from build123d import *

# Parameters (mm, degrees)
IZIM1_W                          = 400
IZIM1_H                          = 400
Y_KSEKLIK_EKSTR_ZYON1_DEPTH      = 30
F_25_5_25_5_AP_DELIK1_AT_2_COUNT = 2
F_25_5_25_5_AP_DELIK1_AT_2_PITCH = 280
F_25_5_25_5_AP_DELIK1_AT_3_COUNT = 2
F_25_5_25_5_AP_DELIK1_AT_3_PITCH = 280
F_25_5_25_5_AP_DELIK1_AT_4_COUNT = 2
F_25_5_25_5_AP_DELIK1_AT_4_PITCH = 395.979797464
KES_EKSTR_ZYON3_DEPTH            = 30
M12_SHCS_IN_HAV_A1_D             = 13
M12_SHCS_IN_HAV_A1_CBORE_D       = 20
M12_SHCS_IN_HAV_A1_CBORE_DEPTH   = 12
M14X2_0_DI_LI_DELIK1_D           = 12
M14X2_0_DI_LI_DELIK1_DEPTH       = 20
M14X2_0_DI_LI_DELIK1_TIP         = 3.605163714


with BuildPart() as part:
    # Çizim1 → Yükseklik-Ekstrüzyon1 (new body)
    with BuildSketch(Plane(origin=(0, 0, 0), x_dir=(1, 0, 0), z_dir=(0, 1, 0))):
        Rectangle(IZIM1_W, IZIM1_H)
    extrude(amount=Y_KSEKLIK_EKSTR_ZYON1_DEPTH)

    # Çizim3 → Ø25.5 (25.5) Çap Delik1 (revolve, cut)
    with BuildSketch(Plane(origin=(-140, 30, 140), x_dir=(0, 0, 1), z_dir=(1, 0, 0))):
        Polygon((0, 0), (0, 30), (20, 30), (12.75, 22.75), (12.75, 7.25), (20, 0), align=None)
    f_25_5_25_5_ap_delik1 = revolve(axis=Axis((-140, 36.35, 140), (0, -1, 0)), mode=Mode.SUBTRACT)

    # Ø25.5 (25.5) Çap Delik1 at 2: Ø25.5 (25.5) Çap Delik1 ×2
    with Locations(*[(0, 0, -i * F_25_5_25_5_AP_DELIK1_AT_2_PITCH) for i in range(1, F_25_5_25_5_AP_DELIK1_AT_2_COUNT)]):
        add(f_25_5_25_5_ap_delik1, mode=Mode.SUBTRACT)

    # Ø25.5 (25.5) Çap Delik1 at 3: Ø25.5 (25.5) Çap Delik1 ×2
    with Locations(*[(i * F_25_5_25_5_AP_DELIK1_AT_3_PITCH, 0, 0) for i in range(1, F_25_5_25_5_AP_DELIK1_AT_3_COUNT)]):
        add(f_25_5_25_5_ap_delik1, mode=Mode.SUBTRACT)

    # Ø25.5 (25.5) Çap Delik1 at 4: Ø25.5 (25.5) Çap Delik1 ×2
    with Locations(*[Vector(0.7071067811865476, 0, -0.7071067811865476) * (i * F_25_5_25_5_AP_DELIK1_AT_4_PITCH) for i in range(1, F_25_5_25_5_AP_DELIK1_AT_4_COUNT)]):
        add(f_25_5_25_5_ap_delik1, mode=Mode.SUBTRACT)

    # Çizim4 → Kes-Ekstrüzyon3 (cut)
    with BuildSketch(Plane(origin=(0, 30, 0), x_dir=(1, 0, 0), z_dir=(0, 1, 0))):
        with BuildLine():
            Line((-15, 49.352110618), (-15, -30.647889382))
            ThreePointArc((-15, -30.647889382), (-35, -50.647889382), (-55, -30.647889382))
            Line((-55, -30.647889382), (-55, 49.352110618))
            ThreePointArc((-55, 49.352110618), (-35, 69.352110618), (-15, 49.352110618))
        make_face()
        with BuildLine():
            Line((55, 49.352110618), (55, -30.647889382))
            ThreePointArc((55, -30.647889382), (35, -50.647889382), (15, -30.647889382))
            Line((15, -30.647889382), (15, 49.352110618))
            ThreePointArc((15, 49.352110618), (35, 69.352110618), (55, 49.352110618))
        make_face()
    extrude(amount=-KES_EKSTR_ZYON3_DEPTH, mode=Mode.SUBTRACT)

    # M12 SHCS İçin Havşa1 (through all)
    with Locations(Plane(origin=(0, 30, 0), x_dir=(1, 0, 0), z_dir=(0, 1, 0))):
        with Locations((-9.135973947, -140.778837954), (-149.99326257, 9.352110618), (-9.135973947, 142.861352041), (143.896335676, 9.352110618)):
            CounterBoreHole(M12_SHCS_IN_HAV_A1_D / 2, M12_SHCS_IN_HAV_A1_CBORE_D / 2, M12_SHCS_IN_HAV_A1_CBORE_DEPTH)

    # M14x2.0 Dişli Delik1
    with Locations(Plane(origin=(0, 30, 0), x_dir=(1, 0, 0), z_dir=(0, 1, 0))):
        with Locations((-96.821851103, -66.289960557)):
            Hole(M14X2_0_DI_LI_DELIK1_D / 2, depth=M14X2_0_DI_LI_DELIK1_DEPTH)
            with Locations((0, 0, -(M14X2_0_DI_LI_DELIK1_DEPTH + M14X2_0_DI_LI_DELIK1_TIP / 2))):  # 118° drill point
                Cone(0, M14X2_0_DI_LI_DELIK1_D / 2, M14X2_0_DI_LI_DELIK1_TIP, mode=Mode.SUBTRACT)


solid = part.part
Source: CAD feature listing. Evaluate the final solid. Frame: model axes, mm. A direction names the side the tool comes from. Give positions to 0.01 mm unless a question says otherwise; leave off trailing zeros. Write each loop counter-clockwise with the first axis right and the second up, starting at its lowest first coordinate (ties: lowest second). Pieces come first, ordered by that corner, then holes. Notation, with made-up numbers: (87.25, -12) - (135.25, -12) arc R32 ccw to (135.25, 23) - close; hole circle Ø1 at (-27.5, 65.5). An arc over 180 degrees is marked (long way). Write item = value, one per line. Start each with the question number.
Q1. Cut plane A-A, the plane x = 35. Return loops of the section in (y, z), then the cut area to 3 significant figures.
Q2. Cut plane B-B, the plane x = -133. Give the number of separate pieces and of enclosed holes in the cut face, then the cut area to 3 significant figures.
Q3. Material intervals for probe 1 along X at (y, z) = (17, -27); probe 2 along X at (y, z) = (19.5, 139.5); probe 3 along Z at (x, y) = (-125.5, 28.5), sorted ascending.
Q4. Reachability of faces 3 (the conical face through (-152.99, 6.9, 138.29)), 4 (the cylindrical face through (-34.56, 15.21, 50.643)), 5 (the cylindrical face through (-92.06, 19.86, 69.94)) from +Z, -Z, +X, -X, +Y, -Y: full face, straight path, thin tool, end or side. Return the list, or none.
Q5. Draft query along Z for faces 1 (the flat face through (-15, 15, -10)), 2 (the flat face through (-3, 15, 200)). Return one class per face: +Z half, -Z half, draft (parallel to the pull), parting line (faces both ways), or undercut.
Computed values:
q1.outline = (0, -200) - (30, -200) - (30, -69.35) - (0, -69.35) - close; (0, 50.65) - (30, 50.65) - (30, 200) - (0, 200) - close
q1.area = 8,400 mm²
q2.separate_pieces = 3
q2.enclosed_holes = 0
q2.area = 10,500 mm²
q3.probe_1 = -200 to -55, -15 to 15, 55 to 200
q3.probe_2 = -200 to -152.74, -127.26 to -19.05, 0.78 to 127.26, 152.74 to 200
q3.probe_3 = -200 to -151.49, -128.51 to 128.51, 151.49 to 200
q4.face_3 = -Y
q4.face_4 = +Y, -Y
q4.face_5 = +Y
q5.face_1 = undercut
q5.face_2 = +Z half
